Answer from the drawing. Dimensions are ordinates in mm from the lowest x, y and z of the part. Coordinates: 2 decimals unless noted, no trailing zeros. Order: outer loops, then holes, each group sorted by start corner. A loop starts at its lowest first (then second) coordinate and runs counter-clockwise, first axis right, second up. Notation, with made-up numbers: (71, 35.25) -> (80, 35.25) arc R15 ccw to (80, 52.25) -> close; hole circle Ø7 at (82, 14.5). An arc over 180 degrees is marked (long way). Answer in a Markdown table with one row per item.
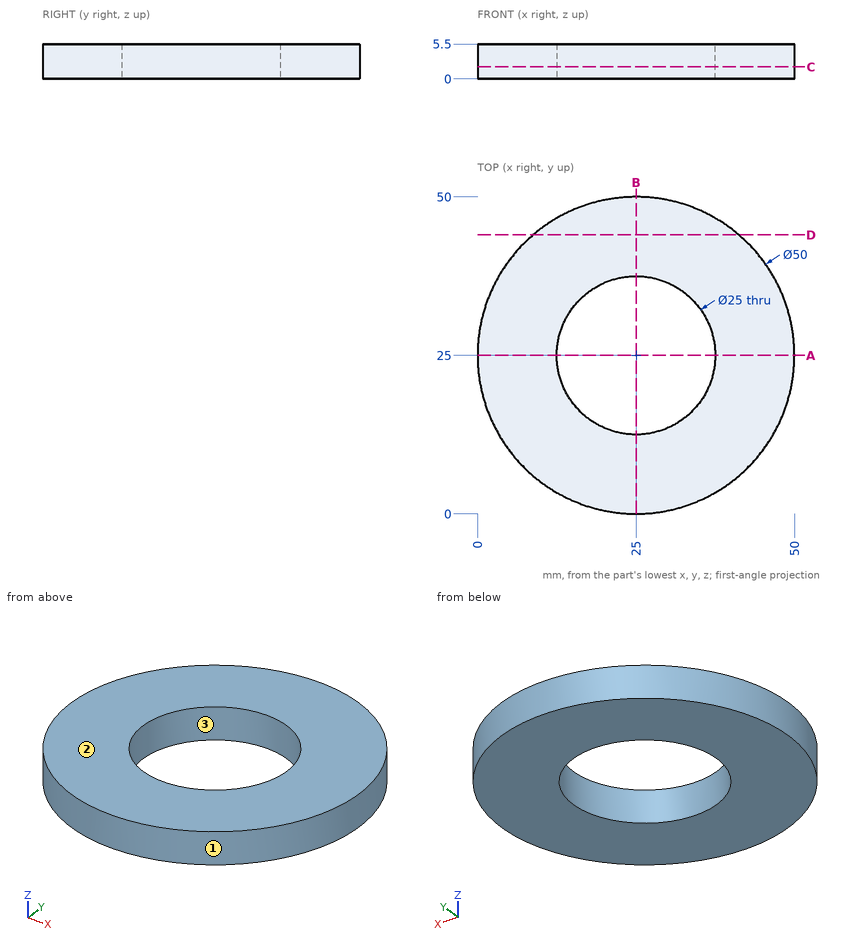
Q1. The part is cut by section A-A (y = 25). Write down the section's boundary in (x, z), then the cut area to 4 significant figures.
Outcome:
| item | result |
|---|---|
| outline | (0, 0) -> (12.5, 0) -> (12.5, 5.5) -> (0, 5.5) -> close; (37.5, 0) -> (50, 0) -> (50, 5.5) -> (37.5, 5.5) -> close |
| area | 137.5 mm² |
Q2. The part is cut by section C-C (z = 1.9). Write down the section's boundary in (x, y), then the cut area to 3 significant figures.
Outcome:
| item | result |
|---|---|
| outline | circle Ø50 at (25, 25); hole circle Ø25 at (25, 25) |
| area | 1,470 mm² |
Q3. Given pin 1 (2 mm diameter, centred on x = 27.5, y = 39.5, fed in from -Z); pin 2 (2 mm diameter, centred on x = 7, z = 3, fed in from -Y), each flat-ended and moving along its own axis, determine where each tip first touches the part or whether it passes through.
Outcome:
| item | result |
|---|---|
| pin 1 | z = 0 |
| pin 2 | y = 6.67 |
Q4. For a pull along X with two mould halves and no side action, classify the marked faces 1, 2 and 3 as pulls with the +X half, pulls with the -X half, needs draft (parallel to the pull), parting line crosses it, or undercut.
Outcome:
| item | result |
|---|---|
| face 1 | parting line crosses it |
| face 2 | needs draft |
| face 3 | undercut |
Q5. Consider line 1 (Y direction, x = 25, z = 3.2); line 2 (X direction, y = 24.5, z = 2.05) (3 decimals); line 3 (Y direction, x = 28, z = 4.5). Determine where each line is inside the solid, lowest interval first.
Outcome:
| item | result |
|---|---|
| line 1 | 0 to 12.5, 37.5 to 50 |
| line 2 | 0.005 to 12.51, 37.49 to 49.995 |
| line 3 | 0.18 to 12.87, 37.13 to 49.82 |
Q6. The part is cut by section D-D (y = 44). Write down the section's boundary in (x, z).
Outcome:
| item | result |
|---|---|
| outline | (8.75, 0) -> (41.25, 0) -> (41.25, 5.5) -> (8.75, 5.5) -> close |
